Design review of the part built by this model. Coordinates are the model's own, in mm. A direction names the side the tool comes from. Coordinates: 2 decimals unless noted, no trailing zeros. Loops run counter-clockwise (first coordinate to the right, second up) from the corner with the lowest first, then second, coordinate; pieces in that order, holes last. Notation, with made-up numbers: M 33.5,-19.5 L 83.5,-19.5 A29 ccw 83.5,1.5 Z; hole C 88,38 d9. An arc over 180 degrees is marked long. Write item = value, one per line. Start each with the question number.
from build123d import *

# Parameters (mm, degrees)
F0_R     = 1.25
F1_DEPTH = 4
F3_DEPTH = 1


with BuildPart() as f1:
    # F0 (on Top) → F1 (new body)
    with BuildSketch(Plane.XY):
        Polygon((20, 0), (28.9777747887, 7.7645713531), (17.3205080757, 10), (21.2132034356, 21.2132034356), (10, 17.3205080757), (7.7645713531, 28.9777747887), (0, 20), (-7.7645713531, 28.9777747887), (-10, 17.3205080757), (-21.2132034356, 21.2132034356), (-17.3205080757, 10), (-28.9777747887, 7.7645713531), (-20, 0), (-28.9777747887, -7.7645713531), (-17.3205080757, -10), (-21.2132034356, -21.2132034356), (-10, -17.3205080757), (-7.7645713531, -28.9777747887), (0, -20), (7.7645713531, -28.9777747887), (10, -17.3205080757), (21.2132034356, -21.2132034356), (17.3205080757, -10), (28.9777747887, -7.7645713531), align=None)
        Circle(F0_R, mode=Mode.SUBTRACT)
        with BuildLine():
            Line((-20, 0), (-28.9777747887, 7.7645713531))
            ThreePointArc((-28.9777747887, 7.7645713531), (-30, 0), (-28.9777747887, -7.7645713531))
            Line((-28.9777747887, -7.7645713531), (-20, 0))
        make_face()
        with BuildLine():
            Line((-17.3205080757, 10), (-21.2132034356, 21.2132034356))
            ThreePointArc((-21.2132034356, 21.2132034356), (-25.9807621135, 15), (-28.9777747887, 7.7645713531))
            Line((-28.9777747887, 7.7645713531), (-17.3205080757, 10))
        make_face()
        with BuildLine():
            Line((-10, 17.3205080757), (-7.7645713531, 28.9777747887))
            ThreePointArc((-7.7645713531, 28.9777747887), (-15, 25.9807621135), (-21.2132034356, 21.2132034356))
            Line((-21.2132034356, 21.2132034356), (-10, 17.3205080757))
        make_face()
        with BuildLine():
            Line((0, 20), (7.7645713531, 28.9777747887))
            ThreePointArc((7.7645713531, 28.9777747887), (0, 30), (-7.7645713531, 28.9777747887))
            Line((-7.7645713531, 28.9777747887), (0, 20))
        make_face()
        with BuildLine():
            Line((10, 17.3205080757), (21.2132034356, 21.2132034356))
            ThreePointArc((21.2132034356, 21.2132034356), (15, 25.9807621135), (7.7645713531, 28.9777747887))
            Line((7.7645713531, 28.9777747887), (10, 17.3205080757))
        make_face()
        with BuildLine():
            Line((17.3205080757, 10), (28.9777747887, 7.7645713531))
            ThreePointArc((28.9777747887, 7.7645713531), (25.9807621135, 15), (21.2132034356, 21.2132034356))
            Line((21.2132034356, 21.2132034356), (17.3205080757, 10))
        make_face()
        with BuildLine():
            ThreePointArc((28.9777747887, -7.7645713531), (29.7433458412, -3.9157857666), (30, 0))
            ThreePointArc((30, 0), (29.7433458412, 3.9157857666), (28.9777747887, 7.7645713531))
            Line((28.9777747887, 7.7645713531), (20, 0))
            Line((20, 0), (28.9777747887, -7.7645713531))
        make_face()
        with BuildLine():
            ThreePointArc((21.2132034356, -21.2132034356), (25.9807621135, -15), (28.9777747887, -7.7645713531))
            Line((28.9777747887, -7.7645713531), (17.3205080757, -10))
            Line((17.3205080757, -10), (21.2132034356, -21.2132034356))
        make_face()
        with BuildLine():
            ThreePointArc((7.7645713531, -28.9777747887), (15, -25.9807621135), (21.2132034356, -21.2132034356))
            Line((21.2132034356, -21.2132034356), (10, -17.3205080757))
            Line((10, -17.3205080757), (7.7645713531, -28.9777747887))
        make_face()
        with BuildLine():
            ThreePointArc((-7.7645713531, -28.9777747887), (0, -30), (7.7645713531, -28.9777747887))
            Line((7.7645713531, -28.9777747887), (0, -20))
            Line((0, -20), (-7.7645713531, -28.9777747887))
        make_face()
        with BuildLine():
            ThreePointArc((-21.2132034356, -21.2132034356), (-15, -25.9807621135), (-7.7645713531, -28.9777747887))
            Line((-7.7645713531, -28.9777747887), (-10, -17.3205080757))
            Line((-10, -17.3205080757), (-21.2132034356, -21.2132034356))
        make_face()
        with BuildLine():
            ThreePointArc((-28.9777747887, -7.7645713531), (-25.9807621135, -15), (-21.2132034356, -21.2132034356))
            Line((-21.2132034356, -21.2132034356), (-17.3205080757, -10))
            Line((-17.3205080757, -10), (-28.9777747887, -7.7645713531))
        make_face()
    extrude(amount=F1_DEPTH)

    # F2 (on face) → F3 (cut)
    with BuildSketch(Plane.XY.offset(4)):
        with BuildLine():
            Line((-24.7956705205, 10.685257294), (-2.5, 3.4409548012))
            Line((-2.5, 3.4409548012), (-2.5, 26.8840101175))
            ThreePointArc((-2.5, 26.8840101175), (-15.8702018119, 21.8434588481), (-24.7956705205, 10.685257294))
        make_face()
        with BuildLine():
            Line((2.5, 26.8840101175), (2.5, 3.4409548012))
            Line((2.5, 3.4409548012), (24.7956705205, 10.685257294))
            ThreePointArc((24.7956705205, 10.685257294), (15.8702018119, 21.8434588481), (2.5, 26.8840101175))
        make_face()
        with BuildLine():
            Line((26.3407554924, 5.9299747125), (4.0450849719, -1.3143277803))
            Line((4.0450849719, -1.3143277803), (17.8245671555, -20.2801579313))
            ThreePointArc((17.8245671555, -20.2801579313), (24.5994239079, -11.1296155999), (27, 0))
            ThreePointArc((27, 0), (26.8346827659, 2.9832534007), (26.3407554924, 5.9299747125))
        make_face()
        with BuildLine():
            Line((13.7794821836, -23.2190841928), (0, -4.2532540418))
            Line((0, -4.2532540418), (-13.7794821836, -23.2190841928))
            ThreePointArc((-13.7794821836, -23.2190841928), (0, -27), (13.7794821836, -23.2190841928))
        make_face()
        with BuildLine():
            Line((-17.8245671555, -20.2801579313), (-4.0450849719, -1.3143277803))
            Line((-4.0450849719, -1.3143277803), (-26.3407554924, 5.9299747125))
            ThreePointArc((-26.3407554924, 5.9299747125), (-25.67852594, -8.3434588481), (-17.8245671555, -20.2801579313))
        make_face()
    extrude(amount=-F3_DEPTH, mode=Mode.SUBTRACT)


solid = f1.part
Q1. Clearance check with flat-ended pins moving along their axes: P1, Ø6.5, axis at x = -13.5, y = 14, coming from the +Z side; P2, Ø0.5, axis at y = 12.5, z = 3.5, coming from the +X side (3 decimals); P3, Ø0.8, axis at y = 9.5, z = 3.5, coming from the -X side. State where each tip first meets the part, or that it passes through.
Q2. Add section B-B on x = -6. State the section outline as (y, z) points.
Q3. For faces 1 (the face through (11, 15, 3)), 2 (the face through (-0.27, -1.22, 1.97)), list the 3-axis set-ups (+Z, -Z, +X, -X, +Y, -Y) from which the entire face can be reached by the end or side of a thin tool; tool diameter is ignored.
Q4. To check wall thickness, follow line 1 (X direction, y = -20, z = 3.5); line 2 (Y direction, x = -17, z = 3.2); line 3 (X direction, y = 11.5, z = 3.3). State the ranges of each line that lie inside material, in increasing order. Write a range as from..to.
Q5. Add section A-A on z = 1.95. State the section outline as (x, y) points, plus the area to 3 significant figures.
Q6. Mouldability with a two-part tool opening along Y and no side actions: class faces 3 (the face through (0, -6, 0)), 4 (the face through (0, -18, 3)) as released by +Y, released by -Y, zero draft, split by the parting line, or undercut.
Q7. Add section D-D on y = 4.5. State the section outline as (x, z) points.
Q8. Add section C-C on y = -14. State the section outline as (x, z) points, plus the area to 3 significant figures.
Values follow:
q1.P1 = 3
q1.P2 = 27.385
q1.P3 = -28.59
q2.outline = M -29.39,0 L 29.39,0 L 29.39,4 L 26.32,4 L 26.32,3 L 4.58,3 L 4.58,4 L -0.68,4 L -0.68,3 L -4.01,3 L -4.01,4 L -12.51,4 L -12.51,3 L -26.32,3 L -26.32,4 L -29.39,4 Z
q3.face_1 = +Z
q3.face_2 = +Z, -Z
q4.line_1 = -22.36..-18.14, -17.62..-11.44, 11.44..17.62, 18.14..22.36
q4.line_2 = -24.72..-19.15, 2.89..8.15, 20.98..24.72
q4.line_3 = -27.71..-24.43, -2.5..2.5, 24.43..27.71
q5.outline = C 0,0 d60; hole C 0,0 d2.5
q5.area = 2,820 mm2
q6.face_3 = zero draft
q6.face_4 = undercut
q7.outline = M -29.66,0 L 29.66,0 L 29.66,4 L 26.62,4 L 26.62,3 L 21.94,3 L 21.94,4 L 5.76,4 L 5.76,3 L 2.5,3 L 2.5,4 L -2.5,4 L -2.5,3 L -5.76,3 L -5.76,4 L -21.94,4 L -21.94,3 L -26.62,3 L -26.62,4 L -29.66,4 Z
q8.outline = M -26.53,0 L 26.53,0 L 26.53,4 L 23.09,4 L 23.09,3 L 13.26,3 L 13.26,4 L 7.08,4 L 7.08,3 L -7.08,3 L -7.08,4 L -13.26,4 L -13.26,3 L -23.09,3 L -23.09,4 L -26.53,4 Z
q8.area = 178 mm2
